Solid Edge part; units mm, degrees
sketch "Sketch1" plane through (0, 0, 0) normal (0, -1, 0) x (1, 0, 0)
  circle A0 centre (0, 0) radius 6.65
extrude "Protrusion1" add sketch "Sketch1" along normal blind 46.2
sketch "Sketch2" plane through (0, -46.2, 0) normal (0, -1, 0) x (1, 0, 0)
  line L0 (-4.1, 4.1) -> (4.1, 4.1)
  line L1 (4.1, 4.1) -> (4.1, -4.1)
  line L2 (4.1, -4.1) -> (-4.1, -4.1)
  line L3 (-4.1, -4.1) -> (-4.1, 4.1)
  dimension "D1" = 4.1
extrude "Cutout1" cut sketch "Sketch2" against normal through all
sketch "Sketch3" plane through (0, 0, 0) normal (0, 1, 0) x (-1, 0, 0)
  line L0 (-3.95, -3.95) -> (-3.95, 3.95)
  line L1 (-3.95, 3.95) -> (3.95, 3.95)
  line L2 (3.95, 3.95) -> (3.95, -3.95)
  line L3 (3.95, -3.95) -> (-3.95, -3.95)
extrude "Protrusion2" add sketch "Sketch3" against normal blind 3
sketch "Sketch4" plane through (0, 0, 0) normal (0, 1, 0) x (-1, 0, 0)
  circle A0 centre (0, 0) radius 6.65
extrude "Extrusionsausprägung_5" add sketch "Sketch4" along normal blind 2
hole "Bohrung_5" at (0, 2, 0) direction (0, -1, 0) diameter 3.5 end up to next
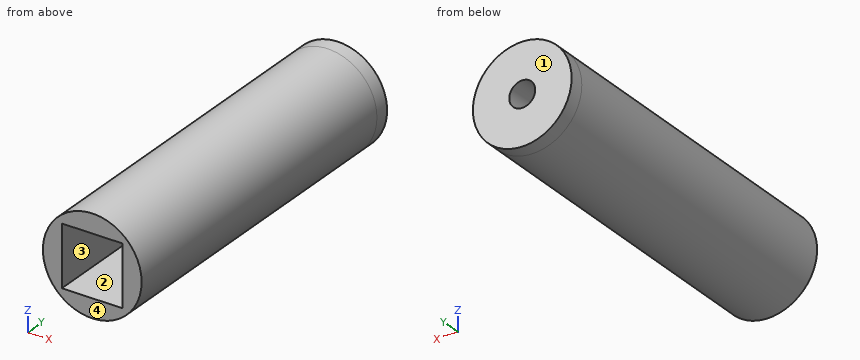
Can you work these out from the model? Positions are in its coordinate system, mm. Face numbers are marked on the shaded views. A direction names the side the tool comes from. Give positions to 0.01 mm unless a question says otherwise; leave off trailing zeros. Loops run counter-clockwise (first coordinate to the right, second up) from the corner with the lowest first, then second, coordinate; pieces in that order, holes last. Notation, with made-up numbers: M 7.25,-36.75 L 22.25,-36.75 A30 cw 22.25,-1.75 Z; hole C 41,61 d4. An arc over 180 degrees is marked long. Use one line per item in the form item = value. Start each with the question number.
(1) I want a section at C-C, the plane x = 1. Write out the boundary of the cut face in (y, z).
(2) I'm going to push flat-ended pins straight in: P1, Ø3, axis at x = 0, z = 0, coming from the -Y side; P2, Ø1.5, axis at x = -1, y = -2, coming from the -Z side; P3, Ø2.5, axis at x = 1.5, y = -1, coming from the +Z side; P4, Ø4, axis at y = -25, z = 2.5, coming from the -X side. Where does each tip first touch, or does it pass through?
(3) On a 3-axis mill with a long thin cutter (end or side, diameter ignored), from which of +Z, -Z, +X, -X, +Y, -Y can I reach the whole of each face in a straight line? I mean the marked faces 3 and 4. Say none if no direction works.
(4) I want a section at A-A, the plane z = 0. Write out the boundary of the cut face in (x, y).
(5) Please list where these lines run through material, in increasing order: line 1 (X direction, y = 0.75, z = 0); line 2 (Z direction, x = 0, y = -27).
(6) I want a section at B-B, the plane y = -0.5. Write out the boundary of the cut face in (x, z).
(7) Thinking about a two-plate mould opening in X: for the marked faces 1 and 2, which applies, released by +X, released by -X, zero draft, split by the parting line, or undercut?
(8) I want a section at D-D, the plane x = -3.25. Write out the boundary of the cut face in (y, z), and give its area (3 significant figures).
Worked out:
q1.outline = M -46.2,-6.57 L 2,-6.57 L 2,-1.44 L -3,-1.44 L -3,-3.95 L 0,-3.95 L 0,-4.1 L -46.2,-4.1 Z; M -46.2,4.1 L 0,4.1 L 0,3.95 L -3,3.95 L -3,1.44 L 2,1.44 L 2,6.57 L -46.2,6.57 Z
q2.P1 = through
q2.P2 = -6.65
q2.P3 = 6.65
q2.P4 = -6.63
q3.face_3 = -Y
q3.face_4 = +Z, -Z, +X, -X, -Y
q4.outline = M -6.65,-46.2 L -4.1,-46.2 L -4.1,0 L -3.95,0 L -3.95,-3 L -1.75,-3 L -1.75,2 L -6.65,2 Z; M 1.75,-3 L 3.95,-3 L 3.95,0 L 4.1,0 L 4.1,-46.2 L 6.65,-46.2 L 6.65,2 L 1.75,2 Z
q5.line_1 = -6.65 to -1.75, 1.75 to 6.65
q5.line_2 = -6.65 to -4.1, 4.1 to 6.65
q6.outline = C 0,0 d13.3; M -3.95,-3.95 L 3.95,-3.95 L 3.95,3.95 L -3.95,3.95 Z; hole M -4.1,-4.1 L 4.1,-4.1 L 4.1,4.1 L -4.1,4.1 Z; hole C 0,0 d3.5
q7.face_1 = zero draft
q7.face_2 = undercut
q8.outline = M -46.2,-5.8 L 2,-5.8 L 2,5.8 L -46.2,5.8 L -46.2,4.1 L 0,4.1 L 0,3.95 L -3,3.95 L -3,-3.95 L 0,-3.95 L 0,-4.1 L -46.2,-4.1 Z
q8.area = 204 mm²
